For this review, take the finished solid that the model builds, in its own axes (mm). A direction names the side the tool comes from. Coordinates: 2 decimals unless noted, no trailing zeros. Write each loop counter-clockwise with the first axis right and the second up, starting at its lowest first coordinate (ties: lowest second). Pieces come first, ordered by that corner, then holes. Notation, with made-up numbers: M 5.25,89 L 16.25,89 A17 ccw 16.25,93 Z; hole C -20,25 d9. An arc over 180 degrees is marked long. One line per question, with ' | ' between items.
from build123d import *

# Parameters (mm, degrees)
SKETCH1_R           = 2
SKETCH1_R_2         = 2.25
BOSS_EXTRUDE1_DEPTH = 4
FILLET2_R           = 1.5
FILLET3_R           = 2
FILLET5_R           = 3
BOSS_EXTRUDE2_DEPTH = 1
CUT_EXTRUDE1_DEPTH  = 2.5
FILLET6_R           = 0.5


with BuildPart() as part:
    # Sketch1 → Boss-Extrude1 (new body)
    with BuildSketch(Plane.XY):
        Polygon((0, 27.5), (0, 46.5), (30, 46.5), (30, 25), (30, 16), (30, 0), (0, 0), (0, 13.5), (4, 13.5), (4, 15), (4, 26), (4, 27.5), align=None)
        with Locations((20, 42.5)):
            Circle(SKETCH1_R, mode=Mode.SUBTRACT)
        with Locations((15, 4)):
            Circle(SKETCH1_R, mode=Mode.SUBTRACT)
        with Locations((10, 42.5)):
            Circle(SKETCH1_R, mode=Mode.SUBTRACT)
        with Locations((3, 42)):
            Circle(SKETCH1_R_2, mode=Mode.SUBTRACT)
        with Locations((27, 42)):
            Circle(SKETCH1_R_2, mode=Mode.SUBTRACT)
    extrude(amount=BOSS_EXTRUDE1_DEPTH)

    # Fillet2
    fillet2_edges = [part.edges().sort_by_distance(p)[0] for p in [
        (0, 27.5, 2),
        (0, 13.5, 2),
    ]]
    fillet(fillet2_edges, radius=FILLET2_R)

    # Fillet3
    fillet3_edges = [part.edges().sort_by_distance(p)[0] for p in [
        (4, 27.5, 2),
        (4, 13.5, 2),
    ]]
    fillet(fillet3_edges, radius=FILLET3_R)

    # Fillet5
    fillet5_edges = [part.edges().sort_by_distance(p)[0] for p in [
        (30, 46.5, 2),
        (30, 0, 2),
        (0, 0, 2),
    ]]
    fillet(fillet5_edges, radius=FILLET5_R)

    # Sketch2 → Boss-Extrude2 (add)
    with BuildSketch(Plane(origin=(0, 0, 0), x_dir=(-1, 0, 0), z_dir=(0, 0, -1))):
        with BuildLine():
            Line((-26, 34.5), (-18.464101615, 34.5))
            ThreePointArc((-18.464101615, 34.5), (-17.464101615, 34.767949192), (-16.732050808, 35.5))
            ThreePointArc((-16.732050808, 35.5), (-15, 36.5), (-13.267949192, 35.5))
            ThreePointArc((-13.267949192, 35.5), (-12.535898385, 34.767949192), (-11.535898385, 34.5))
            Line((-11.535898385, 34.5), (-4, 34.5))
            ThreePointArc((-4, 34.5), (-2, 32.5), (-4, 30.5))
            Line((-4, 30.5), (-26, 30.5))
            ThreePointArc((-26, 30.5), (-28, 32.5), (-26, 34.5))
        make_face()
        with BuildLine():
            Line((-26, 10.5), (-4, 10.5))
            ThreePointArc((-4, 10.5), (-2, 8.5), (-4, 6.5))
            Line((-4, 6.5), (-5.535898385, 6.5))
            ThreePointArc((-5.535898385, 6.5), (-6.535898385, 6.232050808), (-7.267949192, 5.5))
            ThreePointArc((-7.267949192, 5.5), (-9, 4.5), (-10.732050808, 5.5))
            ThreePointArc((-10.732050808, 5.5), (-11.464101615, 6.232050808), (-12.464101615, 6.5))
            Line((-12.464101615, 6.5), (-17.535898385, 6.5))
            ThreePointArc((-17.535898385, 6.5), (-18.535898385, 6.232050808), (-19.267949192, 5.5))
            ThreePointArc((-19.267949192, 5.5), (-21, 4.5), (-22.732050808, 5.5))
            ThreePointArc((-22.732050808, 5.5), (-23.464101615, 6.232050808), (-24.464101615, 6.5))
            Line((-24.464101615, 6.5), (-26, 6.5))
            ThreePointArc((-26, 6.5), (-28, 8.5), (-26, 10.5))
        make_face()
    extrude(amount=BOSS_EXTRUDE2_DEPTH)

    # Sketch3 → Cut-Extrude1 (cut)
    with BuildSketch(Plane(origin=(0, 0, 0), x_dir=(-1, 0, 0), z_dir=(0, 0, -1))):
        Polygon((2.333212821, 27), (-12.5, 27), (-13.618033989, 26.5), (-30, 26.5), (-30, 14.5), (-13.5, 14.5), (-12.499999912, 14), (2.333212821, 14), align=None)
    extrude(amount=-CUT_EXTRUDE1_DEPTH, mode=Mode.SUBTRACT)

    # Fillet6
    fillet6_edges = [part.edges().sort_by_distance(p)[0] for p in [
        (3.322875656, 27, 1.25),
        (3.322875656, 14, 1.25),
        (30, 14.5, 1.25),
        (30, 26.5, 1.25),
    ]]
    fillet(fillet6_edges, radius=FILLET6_R)


solid = part.part
1. Draft analysis for pull direction Y (two halves, no side actions). For faces 5 (the flat face through (22.3, 34.5, -0.5)), 6 (the cylindrical face through (13.4, 2.8, 2)), 7 (the flat face through (4.8, 6.5, -0.5)), state which applies: pulls with the +Y half, pulls with the -Y half, needs draft (parallel to the pull), parting line crosses it, or undercut.
Computed values:
face 5: pulls with the +Y half | face 6: undercut | face 7: pulls with the -Y half
2. Take a section at A-A on z = -0.55. State the section outline as (x, y) points.
Computed values:
outline: M 4,6.5 L 5.54,6.5 A2 cw 7.27,5.5 A2 ccw 10.73,5.5 A2 cw 12.46,6.5 L 17.54,6.5 A2 cw 19.27,5.5 A2 ccw 22.73,5.5 A2 cw 24.46,6.5 L 26,6.5 A2 ccw 26,10.5 L 4,10.5 A2 ccw Z; M 4,30.5 L 26,30.5 A2 ccw 26,34.5 L 18.46,34.5 A2 cw 16.73,35.5 A2 ccw 13.27,35.5 A2 cw 11.54,34.5 L 4,34.5 A2 ccw Z
3. Take a section at C-C on y = 41. State the section outline as (x, z) points.
Computed values:
outline: M 0,0 L 0.98,0 L 0.98,4 L 0,4 Z; M 5.02,0 L 8.68,0 L 8.68,4 L 5.02,4 Z; M 11.32,0 L 18.68,0 L 18.68,4 L 11.32,4 Z; M 21.32,0 L 24.98,0 L 24.98,4 L 21.32,4 Z; M 29.02,0 L 30,0 L 30,4 L 29.02,4 Z
4. Take a section at B-B on x = 20.5. State the section outline as (y, z) points, plus the area to 3 significant figures.
Computed values:
outline: M 0,0 L 4.56,0 L 4.56,-1 L 10.5,-1 L 10.5,0 L 14.5,0 L 14.5,2.5 L 26.5,2.5 L 26.5,0 L 30.5,0 L 30.5,-1 L 34.5,-1 L 34.5,0 L 40.56,0 L 40.56,4 L 0,4 Z; M 44.44,0 L 46.5,0 L 46.5,4 L 44.44,4 Z | area: 150 mm2
5. Clearance check with flat-ended pins moving along their axes: P1, Ø0.8, axis at x = 14, z = -0.5, coming from the -Y side; P2, Ø4, axis at x = 17.5, y = 23.5, coming from the -Z side; P3, Ø0.8, axis at x = 10.5, z = -0.5, coming from the -Y side; P4, Ø1.1, axis at x = 5, z = -0.5, coming from the -Y side. State where each tip first meets the part, or that it passes through.
Computed values:
P1: stops at y = 6.5 | P2: stops at z = 2.5 | P3: stops at y = 4.83 | P4: stops at y = 0
6. Take a section at D-D on z = 3.25. State the section outline as (x, y) points, plus the area to 3 significant figures.
Computed values:
outline: M 0,3 A3 ccw 3,0 L 27,0 A3 ccw 30,3 L 30,43.5 A3 ccw 27,46.5 L 0,46.5 L 0,29 A1.5 ccw 1.5,27.5 L 2,27.5 A2 cw 4,25.5 L 4,15.5 A2 cw 2,13.5 L 1.5,13.5 A1.5 ccw 0,12 Z; hole C 3,42 d4.5; hole C 10,42.5 d4; hole C 15,4 d4; hole C 20,42.5 d4; hole C 27,42 d4.5 | area: 1,260 mm2
7. For line 1 along Y through (x, z) = (27, 1.1); line 2 along Y through (x, z) = (24.5, 2.15); line 3 along Y through (x, z) = (25.25, 2.2), list the stretches that pass through material, from the lowest coordinate up.
Computed values:
line 1: y = 0 to 14.5, 26.5 to 39.75, 44.25 to 46.5 | line 2: y = 0 to 14.5, 26.5 to 46.5 | line 3: y = 0 to 14.5, 26.5 to 40.59, 43.41 to 46.5
8. Machinability: for faces 1 (the flat face through (25.2, 6.5, -0.5)), 2 (the flat face through (15, 6.5, -0.5)), 3 (the flat face through (14.8, 30.5, -0.5)), 4 (the cylindrical face through (2, 32.5, -0.5)), which of the approach directions +Z, -Z, +X, -X, +Y, -Y give a long, thin tool a straight path to every point of the face, cutting with its end or side? Answer none if there is none.
Computed values:
face 1: -Z, +X, -Y | face 2: -Z, -Y | face 3: -Z, +X, -X | face 4: -Z, -X
